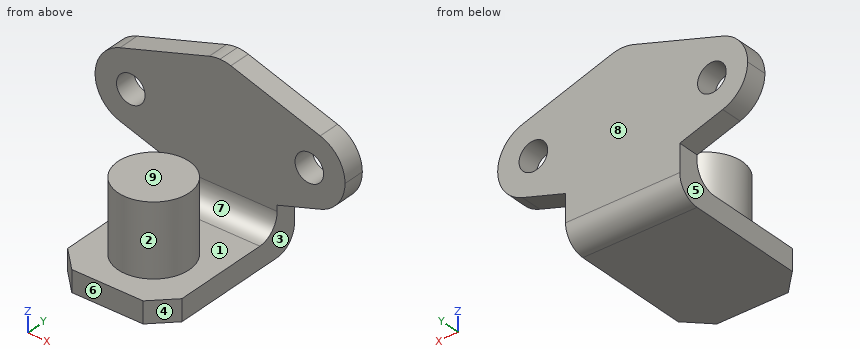
```python
from build123d import *

# Parameters (mm, degrees)
F1_DEPTH = 70
F2_R     = 4
F3_DEPTH = 45.001
F4_R     = 8
F5_DEPTH = 45.001


with BuildPart() as f1:
    # F0 (on Right) → F1 (new body)
    with BuildSketch(Plane.YZ):
        with BuildLine():
            Line((0, 6), (0, 0))
            Line((0, 0), (39, 0))
            ThreePointArc((39, 0), (43.2426406871, 1.7573593129), (45, 6))
            Line((45, 6), (45, 45))
            Line((45, 45), (39, 45))
            Line((39, 45), (39, 12))
            ThreePointArc((39, 12), (37.2426406871, 7.7573593129), (33, 6))
            Line((33, 6), (0, 6))
        make_face()
    extrude(amount=F1_DEPTH)

    # F2 (on Front) → F3 (cut, through all)
    with BuildSketch(Plane.XZ):
        with Locations((10, 27)):
            Circle(F2_R)
        with Locations((60, 27)):
            Circle(F2_R)
        with BuildLine():
            ThreePointArc((63.047757271, 36.524241472), (68.0770530737, 32.8958641135), (70, 27))
            Line((70, 27), (70, 45))
            Line((70, 45), (35, 45))
            ThreePointArc((35, 45), (36.5423335048, 44.880344496), (38.047757271, 44.524241472))
            Line((38.047757271, 44.524241472), (63.047757271, 36.524241472))
        make_face()
        with BuildLine():
            Line((51, 13.620400082), (51, 0))
            Line((51, 0), (70, 0))
            Line((70, 0), (70, 27))
            ThreePointArc((70, 27), (68.0770699689, 21.1041590322), (63.0478118565, 17.4757759955))
            Line((63.0478118565, 17.4757759955), (51, 13.620400082))
        make_face()
        with BuildLine():
            Line((0, 0), (19, 0))
            Line((19, 0), (19, 13.620400082))
            Line((19, 13.620400082), (6.9521881435, 17.4757759955))
            ThreePointArc((6.9521881435, 17.4757759955), (1.922930031, 21.1041590323), (0, 27.0000000001))
            Line((0, 27.0000000001), (0, 0))
        make_face()
        with BuildLine():
            Line((0, 45), (0, 27.0000000001))
            ThreePointArc((0, 27.0000000001), (1.9229469263, 32.8958641136), (6.952242729, 36.524241472))
            Line((6.952242729, 36.524241472), (31.952242729, 44.524241472))
            ThreePointArc((31.952242729, 44.524241472), (33.4576664952, 44.880344496), (35, 45))
            Line((35, 45), (0, 45))
        make_face()
    extrude(amount=-F3_DEPTH, mode=Mode.SUBTRACT)

    # F4 (on Top) → F5 (cut, through all)
    with BuildSketch(Plane.XY):
        with Locations((35, 16)):
            Circle(F4_R)
        Polygon((19, 0), (25, 0), (19, 6), align=None)
        Polygon((45, 0), (51, 0), (51, 6), align=None)
    extrude(amount=F5_DEPTH, mode=Mode.SUBTRACT)

    # F7 (on offset) → F8 (revolve)
    with BuildSketch(Plane.XZ.offset(-16)):
        Polygon((35, 26), (35, 0), (43, 0), (43, 6), (45, 6), (45, 26), align=None)
    revolve(axis=Axis((35, 16, 13), (0, 0, 1)))


solid = f1.part
```
Geometry: final body of the model. Coordinates: model frame, mm. Face numbers are marked on the shaded views. A direction names the side the tool comes from. Coordinates: 2 decimals unless noted, no trailing zeros. Order: outer loops, then holes, each group sorted by start corner. A loop starts at its lowest first (then second) coordinate and runs counter-clockwise, first axis right, second up. Notation, with made-up numbers: (48, 55) - (72, 55) arc R30 ccw to (72, 91) - close; hole circle Ø2 at (-34.75, -21.5). An arc over 180 degrees is marked (long way). Return JSON: item names as keys, results as strings. Group by question number.
1. Cut plane B-B (x = 60). Output: boundary loops of the cut face in (y, z), plus the area to 3 significant figures.
2. Cut plane A-A (z = 19). Output: boundary loops of the cut face in (x, y), plus the area to 3 significant figures.
3. Cut plane D-D (z = 24.5). Output: boundary loops of the cut face in (x, y).
4. Material intervals for line 1 along Y through (x, z) = (61, 31.5); line 2 along X through (y, z) = (17, 4); line 3 along Z through (x, y) = (24, 28.5), sorted ascending. Write a range as [from, to].
5. Set-up query: the marked faces 5, 6, 7, 8 and 9. Return all of +Z, -Z, +X, -X, +Y, -Y with unobstructed straight access to the full face (end or side cutting, diameter ignored); none if empty.
6. Pin query (flat end, axial travel): pin 1 (10 mm diameter, centred on x = 43.5, z = 24, fed in from -Y); pin 2 (11 mm diameter, centred on y = 29.5, z = 5, fed in from -X); pin 3 (2 mm diameter, centred on x = 46, y = 6, fed in from +Z). Return the tip coordinate at first contact, or that it passes through.
7. Cut plane C-C (y = 41.5). Output: boundary loops of the cut face in (x, z).
8. Pull-direction query (Y, two-part tool) for the marked faces 1, 2, 3 and 4; classes: pulls with the +Y half, pulls with the -Y half, needs draft (parallel to the pull), parting line crosses it, or undercut.
Resolved:
{
 "1": {"outline": "(39, 16.5) - (45, 16.5) - (45, 23) - (39, 23) - close; (39, 31) - (45, 31) - (45, 37.5) - (39, 37.5) - close", "area": "78.0 mm²"},
 "2": {"outline": "(4, 39) - (66, 39) - (66, 45) - (4, 45) - close; circle Ø20 at (35, 16)", "area": "686 mm²"},
 "3": {"outline": "(0.32, 39) - (6.88, 39) - (6.88, 45) - (0.32, 45) - close; (13.12, 39) - (56.88, 39) - (56.88, 45) - (13.12, 45) - close; circle Ø20 at (35, 16); (63.12, 39) - (69.68, 39) - (69.68, 45) - (63.12, 45) - close"},
 "4": {"line 1": "y = [39, 45]", "line 2": "x = [19, 51]", "line 3": "z = [0, 6]"},
 "5": {"face 5": "-Z, -X, +Y, -Y", "face 6": "+Z, -Z, +X, -X, -Y", "face 7": "+Z, +X, -X", "face 8": "+Z, -Z, +X, -X, +Y", "face 9": "+Z, +X, -X, -Y"},
 "6": {"pin 1": "stops at y = 6.63", "pin 2": "stops at x = 19", "pin 3": "stops at z = 6"},
 "7": {"outline": "(6.95, 17.48) - (19, 13.62) - (19, 0.55) - (51, 0.55) - (51, 13.62) - (63.05, 17.48) arc R10 ccw to (63.05, 36.52) - (38.05, 44.52) arc R10 ccw to (31.95, 44.52) - (6.95, 36.52) arc R10 ccw to start; hole circle Ø8 at (10, 27); hole circle Ø8 at (60, 27)"},
 "8": {"face 1": "undercut", "face 2": "undercut", "face 3": "needs draft", "face 4": "pulls with the -Y half"}
}
